The listing builds one solid part. Answer for the finished solid, in the listing's coordinates (mm). Give positions to 0.01 mm unless a question says otherwise; leave off trailing zeros. Loops run counter-clockwise (first coordinate to the right, second up) from the corner with the lowest first, then second, coordinate; pieces in that order, holes last.
Item 1: Section A-A, the plane y = -4.5 is taken. Give the vertices of the cut face in (x, z), and give its area (3 significant figures).
Item 2: Each of these flat-tipped pins is pushed along its axis until it touches: pin 1 Ø4 at (x, y) = (47.5, -3) entering from +Z; pin 2 Ø1 at (y, z) = (-3, 57) entering from -X; pin 3 Ø3 at (x, y) = (62.5, -0.5) entering from +Z. Where does it stop, or does it pass through?
Item 3: Consider line 1 along X through (y, z) = (0.5, -41); line 2 along Z through (x, y) = (59.5, -1.75); line 3 along Z through (x, y) = (-79, -4.25). Determine where each line is inside the solid, lowest interval first.
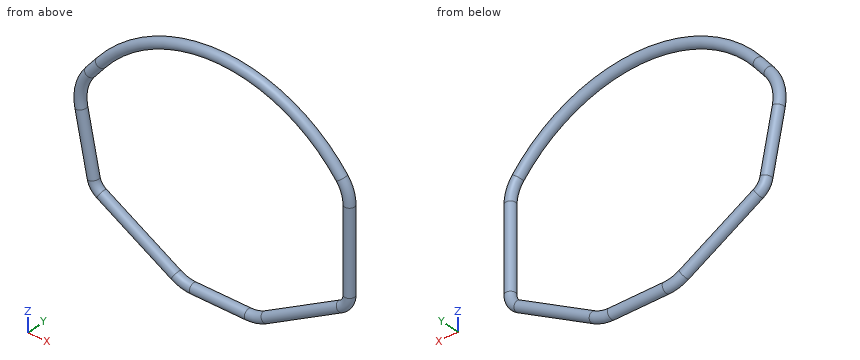
from build123d import *

# Parameters (mm, degrees)
SKETCH2_R = 3.4925


with BuildPart() as part:
    # Sweep1: sweep along a path in Sketch1
    with BuildLine(Plane(origin=(0, -2.640079968, 0), x_dir=(-1, 0, 0), z_dir=(0, -1, 0))) as sweep1_path:
        Line((83.350830382, -38.950762016), (90.921866986, -29.516691169))
        ThreePointArc((90.921866986, -29.516691169), (96.854212201, -17.461644901), (97.114610152, -4.028512237))
        Line((97.114610152, -4.028512237), (88.555415825, 38.286098976))
        ThreePointArc((88.555415825, 38.286098976), (86.599981286, 42.766938519), (82.974870066, 46.04721532))
        Line((82.974870066, 46.04721532), (31.21997499, 75.927917924))
        ThreePointArc((31.21997499, 75.927917924), (25.353847026, 78.357747685), (19.058716307, 79.186517367))
        Line((19.058716307, 79.186517367), (-19.058716307, 79.186517367))
        ThreePointArc((-19.058716307, 79.186517367), (-25.353847026, 78.357747685), (-31.21997499, 75.927917924))
        Line((-31.21997499, 75.927917924), (-83.485748808, 45.752259341))
        ThreePointArc((-83.485748808, 45.752259341), (-87.73988542, 41.498122729), (-89.297007491, 35.686864045))
        Line((-89.297007491, 35.686864045), (-89.297007491, -22.979722438))
        ThreePointArc((-89.297007491, -22.979722438), (-87.965976384, -30.91549024), (-84.118562377, -37.98270043))
        ThreePointArc((-84.118562377, -37.98270043), (-0.617769304, -78.930731865), (83.350830382, -38.950762016))
    # Sketch2 → Sweep1 (sweep)
    with BuildSketch(Plane(origin=(0, 0, 0), x_dir=(0, 0, -1), z_dir=(1, 0, 0))):
        with Locations((79.186517367, -2.640079968)):
            Circle(SKETCH2_R)
    sweep(path=sweep1_path.line)


solid = part.part
Worked answers:
1. outline: (-100.01, 3.44) - (-91.45, -38.87) arc R14.58 ccw to (-84.45, -48.61) - (-32.7, -78.49) arc R27.28 ccw to (-19.06, -82.14) - (19.06, -82.14) arc R27.28 ccw to (32.7, -78.49) - (84.96, -48.31) arc R14.58 ccw to (92.25, -35.69) - (92.25, 22.98) arc R27.28 ccw to (86.45, 39.81) arc R109.83 ccw to (-85.66, 40.8) - (-93.23, 31.37) arc R33.88 ccw to start; hole (-94.22, 4.61) - (-85.66, -37.7) arc R8.67 ccw to (-81.5, -43.49) - (-29.74, -73.37) arc R21.37 ccw to (-19.06, -76.23) - (19.06, -76.23) arc R21.37 ccw to (29.74, -73.37) - (82.01, -43.19) arc R8.67 ccw to (86.34, -35.69) - (86.34, 22.98) arc R21.37 ccw to (81.79, 36.16) arc R103.92 ccw to (-81.05, 37.1) - (-88.62, 27.67) arc R27.97 ccw to start
1. area: 3,280 mm2
2. pin 1: stops at z = 72.6
2. pin 2: stops at x = -71.04
2. pin 3: stops at z = 63.56
3. line 1: x = -89.32 to -85.92, 86.26 to 89.7
3. line 2: z = -63.5 to -55.7, 56.74 to 64.88
3. line 3: z = -51.92 to -44.76, 39.35 to 48.56
